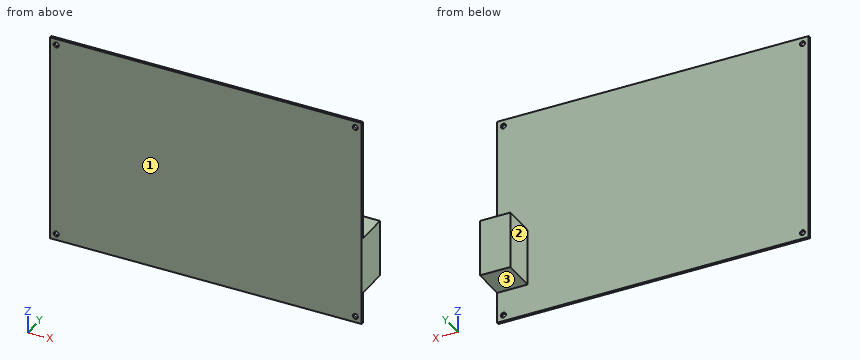
from build123d import *

# Parameters (mm, degrees)
SKETCH1_W           = 200
SKETCH1_H           = 135
SKETCH1_R           = 1.65
BOSS_EXTRUDE1_DEPTH = 1.6
SKETCH2_W           = 36.6
SKETCH2_H           = 21.25
BOSS_EXTRUDE2_DEPTH = 19.5


with BuildPart() as part:
    # Sketch1 → Boss-Extrude1 (new body)
    with BuildSketch(Plane(origin=(0, 0, 0), x_dir=(1, 0, 0), z_dir=(0, 1, 0))):
        with Locations((100, 67.5)):
            Rectangle(SKETCH1_W, SKETCH1_H)
        with Locations(Location((196, 131, 0), (0, 0, 270))):
            Circle(SKETCH1_R, mode=Mode.SUBTRACT)
        with Locations(Location((4, 131, 0), (0, 0, 90))):
            Circle(SKETCH1_R, mode=Mode.SUBTRACT)
        with Locations(Location((4, 4, 0), (0, 0, 270))):
            Circle(SKETCH1_R, mode=Mode.SUBTRACT)
        with Locations(Location((196, 4, 0), (0, 0, 90))):
            Circle(SKETCH1_R, mode=Mode.SUBTRACT)
    extrude(amount=BOSS_EXTRUDE1_DEPTH)

    # Sketch2 → Boss-Extrude2 (add)
    with BuildSketch(Plane(origin=(200, 0, 0), x_dir=(0, 0, -1), z_dir=(1, 0, 0))):
        with Locations((96.7, 12.225)):
            Rectangle(SKETCH2_W, SKETCH2_H)
    extrude(amount=-BOSS_EXTRUDE2_DEPTH)


solid = part.part
Could you check a few things on this model? Use its own coordinates, in mm. Face numbers are marked on the shaded views. A direction names the side the tool comes from. Give positions to 0.01 mm unless a question says otherwise; leave off trailing zeros. Order: outer loops, then holes, each group sorted by start corner. A loop starts at its lowest first (then second) coordinate and runs counter-clockwise, first axis right, second up.
Item 1: If we section it at C-C, the plane y = 7.75: Write out the boundary of the cut face in (x, z), plus the area to 3 significant figures.
Item 2: For the marked faces 1, 2 and 3, which set-ups out of +Z, -Z, +X, -X, +Y, -Y let a thin tool reach every point of the face, with its end or its side?
Item 3: I'm going to push a flat-ended pin straight in: pin 1 (4 mm diameter, centred on x = 112, z = -47, fed in from +Y). Where does the tip first touch, or does it pass through?
Item 4: If we section it at B-B, the plane x = 76.5: Write out the boundary of the cut face in (y, z), plus the area to 3 significant figures.
Item 5: If we section it at A-A, the plane z = -106.5: Write out the boundary of the cut face in (x, y).
Item 6: I need wall thicknesses on line 1 (X direction, y = 0.4, z = -4); line 2 (Z direction, x = 196, y = 0.3); line 3 (Y direction, x = 129, z = -112.5). Which ranges of each line are inside material? Lowest first, please.
Values:
1. outline: (180.5, -115) - (200, -115) - (200, -78.4) - (180.5, -78.4) - close
1. area: 714 mm2
2. face 1: +Z, -Z, +X, -X, -Y
2. face 2: +Z, -Z, -X, +Y
2. face 3: -Z, +X, -X, +Y
3. pin 1: stops at y = 1.6
4. outline: (0, -135) - (1.6, -135) - (1.6, 0) - (0, 0) - close
4. area: 216 mm2
5. outline: (0, 0) - (200, 0) - (200, 22.85) - (180.5, 22.85) - (180.5, 1.6) - (0, 1.6) - close
6. line 1: x = 0 to 2.35, 5.65 to 194.35, 197.65 to 200
6. line 2: z = -135 to -132.65, -129.35 to -5.65, -2.35 to 0
6. line 3: y = 0 to 1.6
